```python
from build123d import *

# Parameters (mm, degrees)
SKETCH1_W           = 49
SKETCH1_H           = 10
SKETCH1_R           = 2.15
SKETCH1_R_2         = 2.175
SKETCH1_R_3         = 2.2
SKETCH1_R_4         = 2.225
SKETCH1_R_5         = 2.3
SKETCH1_R_6         = 2.25
SKETCH1_R_7         = 2.275
BOSS_EXTRUDE1_DEPTH = 8
FILLET1_R           = 2


with BuildPart() as part:
    # Sketch1 → Boss-Extrude1 (new body)
    with BuildSketch(Plane(origin=(0, 0, 0), x_dir=(1, 0, 0), z_dir=(0, 1, 0))):
        with Locations((24.5, 5)):
            Rectangle(SKETCH1_W, SKETCH1_H)
        with Locations(Location((5, 5, 0), (0, 0, 270))):
            Circle(SKETCH1_R, mode=Mode.SUBTRACT)
        with Locations(Location((11.5, 5, 0), (0, 0, 270))):
            Circle(SKETCH1_R_2, mode=Mode.SUBTRACT)
        with Locations(Location((18, 5, 0), (0, 0, 270))):
            Circle(SKETCH1_R_3, mode=Mode.SUBTRACT)
        with Locations(Location((24.5, 5, 0), (0, 0, 270))):
            Circle(SKETCH1_R_4, mode=Mode.SUBTRACT)
        with Locations(Location((44, 5, 0), (0, 0, 270))):
            Circle(SKETCH1_R_5, mode=Mode.SUBTRACT)
        with Locations(Location((31, 5, 0), (0, 0, 270))):
            Circle(SKETCH1_R_6, mode=Mode.SUBTRACT)
        with Locations(Location((37.5, 5, 0), (0, 0, 270))):
            Circle(SKETCH1_R_7, mode=Mode.SUBTRACT)
    extrude(amount=BOSS_EXTRUDE1_DEPTH)

    # Fillet1
    fillet1_edges = [part.edges().sort_by_distance(p)[0] for p in [
        (0, 4, -10),
        (49, 4, -10),
        (49, 4, 0),
        (0, 4, 0),
    ]]
    fillet(fillet1_edges, radius=FILLET1_R)


solid = part.part
```
Model file for the job. Use its own axes, mm. Round coordinates to 2 decimals unless told otherwise and drop trailing zeros. Write each loop counter-clockwise with the first axis right and the second up, starting at its lowest first coordinate (ties: lowest second). Pieces come first, ordered by that corner, then holes. Notation, with made-up numbers: (-28.5, 58) - (18.5, 58) arc R30 ccw to (18.5, 92) - close; hole circle Ø1 at (27.25, -20.75). An arc over 180 degrees is marked (long way). One line per item, written item: value.
(1) Two-plate mould, pull along X, no slides. Class faces 1 (the cylindrical face through (5.09, 3.94, -7.15)), 2 (the cylindrical face through (0.57, 4.06, -9.4)), 3 (the cylindrical face through (48.4, 4.06, -0.57)): pulls with the +X half, pulls with the -X half, needs draft (parallel to the pull), parting line crosses it, or undercut.
Values follow:
face 1: undercut
face 2: pulls with the -X half
face 3: pulls with the +X half
(2) Drop a flat-ended pin along its axis: P1, Ø2.5, axis at x = 5, z = -5, coming from the +Y side. Give the stop position or say it passes through.
Values follow:
P1: passes through
(3) Cut at B-B, the plane z = -6.25. Give the number of separate pieces and of enclosed holes in the cut face, plus the area to 3 significant figures.
Values follow:
separate pieces: 8
enclosed holes: 0
area: 186 mm²
(4) Wall check: probe 1 along Z at (x, y) = (13.5, 3.5); probe 2 along Z at (x, y) = (32.5, 7); probe 3 along X at (y, z) = (4.5, -9.5). Give the ranges that are in metal, low to high.
Values follow:
probe 1: z = -10 to -5.85, -4.15 to 0
probe 2: z = -10 to -6.68, -3.32 to 0
probe 3: x = 0.68 to 48.32
(5) Cut at C-C, the plane y = 3.75. Give the cut face in (x, z) (3 decimals).
Values follow:
outline: (0, -8) arc R2 ccw to (2, -10) - (47, -10) arc R2 ccw to (49, -8) - (49, -2) arc R2 ccw to (47, 0) - (2, 0) arc R2 ccw to (0, -2) - close; hole circle Ø4.3 at (5, -5); hole circle Ø4.35 at (11.5, -5); hole circle Ø4.4 at (18, -5); hole circle Ø4.45 at (24.5, -5); hole circle Ø4.5 at (31, -5); hole circle Ø4.55 at (37.5, -5); hole circle Ø4.6 at (44, -5)
(6) Cut at A-A, the plane x = 11.5. Give the cut face in (y, z) (3 decimals), plus the area to 3 significant figures.
Values follow:
outline: (0, -10) - (8, -10) - (8, -7.175) - (0, -7.175) - close; (0, -2.825) - (8, -2.825) - (8, 0) - (0, 0) - close
area: 45.2 mm²
(7) Cut at D-D, the plane x = 5. Give the cut face in (y, z), plus the area to 3 significant figures.
Values follow:
outline: (0, -10) - (8, -10) - (8, -7.15) - (0, -7.15) - close; (0, -2.85) - (8, -2.85) - (8, 0) - (0, 0) - close
area: 45.6 mm²
